```python
from build123d import *

# Parameters (mm, degrees)
SKETCH_1_W      = 56
SKETCH_1_H      = 15
SKETCH_1_R      = 1.7
EXTRUDE_1_DEPTH = 23
CHAMFER_2_SIZE  = 7
FILLET_1_R      = 3


with BuildPart() as part:
    # 草图1 → 凸台-拉伸1 (new body)
    with BuildSketch(Plane.XY):
        Rectangle(SKETCH_1_W, SKETCH_1_H)
        with Locations((22, 0)):
            Circle(SKETCH_1_R, mode=Mode.SUBTRACT)
        with Locations((-22, 0)):
            Circle(SKETCH_1_R, mode=Mode.SUBTRACT)
    extrude(amount=EXTRUDE_1_DEPTH)

    # 倒角2
    chamfer_2_edges = [part.edges().sort_by_distance(p)[0] for p in [
        (28, -7.5, 11.5),
        (-28, -7.5, 11.5),
    ]]
    chamfer(chamfer_2_edges, length=CHAMFER_2_SIZE)

    # 圆角1
    fillet_1_edges = [part.edges().sort_by_distance(p)[0] for p in [
        (28, -0.5, 11.5),
        (-21, -7.5, 11.5),
        (21, -7.5, 11.5),
        (-28, -0.5, 11.5),
        (-28, 7.5, 11.5),
        (28, 7.5, 11.5),
    ]]
    fillet(fillet_1_edges, radius=FILLET_1_R)


solid = part.part
```
Work out the finished part from the listing and answer in its coordinate system (mm). Give positions to 0.01 mm unless a question says otherwise; leave off trailing zeros. Order: outer loops, then holes, each group sorted by start corner. A loop starts at its lowest first (then second) coordinate and runs counter-clockwise, first axis right, second up. Notation, with made-up numbers: (1.25, 8) - (60.25, 8) arc R15 cw to (60.25, 19) - close; hole circle Ø7 at (43.25, -9). An arc over 180 degrees is marked (long way). One line per item, written item: value. Start each with the question number.
1. Section B-B, the plane y = 0 is taken. Write down the section's boundary in (x, z), then the cut area to 3 significant figures.
2. For a pull along X with two mould halves and no side action, classify faces 1 (the face through (28, 3, 11)), 2 (the face through (-20.921, -7.265, 11.661)), 3 (the face through (-20.43, -0.65, 11.34)) as released by +X, released by -X, zero draft, split by the parting line, or undercut.
3. Each of these flat-tipped pins is pushed along its axis until it touches: pin 1 Ø2.5 at (x, y) = (-22, 0) entering from -Z; pin 2 Ø3 at (y, z) = (-4, 19.5) entering from +X; pin 3 Ø1 at (y, z) = (-4.5, 14) entering from -X. Where does it stop, or does it pass through?
4. Section A-A, the plane z = 11 is taken. Write down the section's boundary in (x, y), then the cut area to 3 significant figures.
5. Consider line 1 (Y direction, x = -22, z = 15.25); line 2 (Y direction, x = -21, z = 11.75); line 3 (X direction, y = -3.5, z = 11.5). Determine where each line is inside the solid, lowest interval first.
6. Section C-C, the plane y = -3.5 is taken. Write down the section's boundary in (x, z).
Filled sheet:
1. outline: (-27.91, 0) - (-23.7, 0) - (-23.7, 23) - (-27.91, 23) - close; (-20.3, 0) - (20.3, 0) - (20.3, 23) - (-20.3, 23) - close; (23.7, 0) - (27.91, 0) - (27.91, 23) - (23.7, 23) - close
1. area: 1,130 mm²
2. face 1: released by +X
2. face 2: released by -X
2. face 3: undercut
3. pin 1: through
3. pin 2: x = 26
3. pin 3: x = -24.5
4. outline: (-28, 0.74) arc R3 ccw to (-27.12, -1.38) - (-21.88, -6.62) arc R3 ccw to (-19.76, -7.5) - (19.76, -7.5) arc R3 ccw to (21.88, -6.62) - (27.12, -1.38) arc R3 ccw to (28, 0.74) - (28, 4.5) arc R3 ccw to (25, 7.5) - (-25, 7.5) arc R3 ccw to (-28, 4.5) - close; hole circle Ø3.4 at (-22, 0); hole circle Ø3.4 at (22, 0)
4. area: 768 mm²
5. line 1: -6.5 to -1.7, 1.7 to 7.5
5. line 2: -7.23 to -1.37, 1.37 to 7.5
5. line 3: -25 to 25
6. outline: (-25, 0) - (25, 0) - (25, 23) - (-25, 23) - close
